Can you work these out from the model? Positions are in its coordinate system, mm. A direction names the side the tool comes from. Round coordinates to 2 decimals unless told otherwise and drop trailing zeros. Write each loop counter-clockwise with the first axis right and the second up, starting at its lowest first coordinate (ties: lowest second). Pieces come first, ordered by that corner, then holes.
Q1. We'd pull the mould along X, two halves only. Please class faces 5 (the cylindrical face through (1.4, -13.294, 613.956)), 6 (the flat face through (-70, 105, 629)), 7 (the flat face through (-50, 105, 629)): +X half, -X half, draft (parallel to the pull), parting line (faces both ways), or undercut.
Q2. I'm going to push flat-ended pins straight in: pin 1 Ø6 at (x, z) = (-34.5, 194) entering from +Y; pin 2 Ø20.5 at (x, y) = (-35, -665.5) entering from -Z; pin 3 Ø1 at (x, z) = (17.5, 164.5) entering from -Y; pin 4 Ø23.5 at (x, y) = (35, 665.5) entering from +Z. Where does each tip first touch, or does it pass through?
Q3. Please list where these lines run through material, in increasing order: line 1 along X through (y, z) = (-665.5, 37.75); line 2 along Y through (x, z) = (35, 29); line 3 along Y through (x, z) = (-35, 32).
Q4. If we section it at C-C (y = 373): Please give me the cut outline in (x, z), plus the area to 3 significant figures.
Q5. For faces 1 (the flat face through (50, -105, 629)), 2 (the flat face through (-1, 664, 45)), 3 (the flat face through (70, -105, 629)), 4 (the cylindrical face through (-84.79, 13.31, 633.96)), which set-ups out of +Z, -Z, +X, -X, +Y, -Y let a thin tool reach every point of the face, with its end or its side?
Q6. If we section it at B-B (z = 216): Please give me the cut outline in (x, y).
Q7. If we section it at D-D (z = 82.5): Please give me the cut outline in (x, y).
from build123d import *

# Parameters (mm, degrees)
F1_DEPTH  = 100
F4_DEPTH  = 20
F7_DEPTH  = 20
F8_W      = 200
F8_H      = 81.5832222524
F9_DEPTH  = 30
F10_R     = 9
F11_DEPTH = 672.101


with BuildPart() as f1:
    # F0 (on Right) → F1 (new body, symmetric)
    with BuildSketch(Plane.YZ):
        with BuildLine():
            ThreePointArc((-613.9167777476, 15), (0, 614.1), (613.9167777476, 15))
            Line((613.9167777476, 15), (633.9225583618, 15))
            ThreePointArc((633.9225583618, 15), (0, 634.1), (-633.9225583618, 15))
            Line((-633.9225583618, 15), (-613.9167777476, 15))
        make_face()
    extrude(amount=F1_DEPTH, both=True)

    # F3 (on offset) → F4 (join)
    with BuildSketch(Plane.YZ.offset(70)):
        with BuildLine():
            ThreePointArc((-633.9225583618, 15), (0, 634.1), (633.9225583618, 15))
            Line((633.9225583618, 15), (686.9362488616, 15))
            ThreePointArc((686.9362488616, 15), (0, 687.1), (-686.9362488616, 15))
            Line((-686.9362488616, 15), (-633.9225583618, 15))
        make_face()
    extrude(amount=-F4_DEPTH)

    # F6 (on offset) → F7 (join)
    with BuildSketch(Plane(origin=(-70, 0, 0), x_dir=(0, -1, 0), z_dir=(-1, 0, 0))):
        with BuildLine():
            Line((-686.9362488616, 15), (-633.9225583618, 15))
            ThreePointArc((-633.9225583618, 15), (0, 634.1), (633.9225583618, 15))
            Line((633.9225583618, 15), (686.9362488616, 15))
            ThreePointArc((686.9362488616, 15), (0, 687.1), (-686.9362488616, 15))
        make_face()
    extrude(amount=-F7_DEPTH)

    # F8 (on face) → F9 (join)
    with BuildSketch(Plane(origin=(0, 0, 15), x_dir=(1, 0, 0), z_dir=(0, 0, -1))):
        with Locations((0, -654.7083888738)):
            Rectangle(F8_W, F8_H)
        Polygon((-100, 695.5), (-100, 633.9225583618), (-70, 633.9225583618), (-70, 686.9362488616), (-50, 686.9362488616), (-50, 633.9225583618), (50, 633.9225583618), (50, 686.9362488616), (70, 686.9362488616), (70, 633.9225583618), (100, 633.9225583618), (100, 695.5), align=None)
        Polygon((-100, 633.9225583618), (-100, 613.9167777476), (100, 613.9167777476), (100, 633.9225583618), (70, 633.9225583618), (70, 686.9362488616), (50, 686.9362488616), (50, 633.9225583618), (-50, 633.9225583618), (-50, 686.9362488616), (-70, 686.9362488616), (-70, 633.9225583618), align=None)
    extrude(amount=-F9_DEPTH)

    # F10 (on face) → F11 (cut, through all)
    with BuildSketch(Plane(origin=(0, 0, 15), x_dir=(1, 0, 0), z_dir=(0, 0, -1))):
        with Locations((-35, 665.5)):
            Circle(F10_R)
        with Locations((35, 665.5)):
            Circle(F10_R)
        with Locations((-35, -665.5)):
            Circle(F10_R)
        with Locations((35, -665.5)):
            Circle(F10_R)
    extrude(amount=-F11_DEPTH, mode=Mode.SUBTRACT)


solid = f1.part
A:
1. face 5: draft
1. face 6: -X half
1. face 7: undercut
2. pin 1: stops at y = 604.65
2. pin 2: stops at z = 15
2. pin 3: stops at y = -612.52
2. pin 4: stops at z = 45
3. line 1: x = -100 to -44, -26 to 26, 44 to 100
3. line 2: y = -695.5 to -674.5, -656.5 to -613.41, 613.41 to 656.5, 674.5 to 695.5
3. line 3: y = -695.5 to -674.5, -656.5 to -613.27, 613.27 to 656.5, 674.5 to 695.5
4. outline: (-100, 487.84) - (100, 487.84) - (100, 512.79) - (70, 512.79) - (70, 577.04) - (50, 577.04) - (50, 512.79) - (-50, 512.79) - (-50, 577.04) - (-70, 577.04) - (-70, 512.79) - (-100, 512.79) - close
4. area: 7,560 mm2
5. face 1: +Z
5. face 2: +Z, +Y
5. face 3: +Z, +X
5. face 4: +Z, -X
6. outline: (-100, -596.18) - (-70, -596.18) - (-70, -652.27) - (-50, -652.27) - (-50, -596.18) - (50, -596.18) - (50, -652.27) - (70, -652.27) - (70, -596.18) - (100, -596.18) - (100, -574.86) - (-100, -574.86) - close; (-100, 574.86) - (100, 574.86) - (100, 596.18) - (70, 596.18) - (70, 652.27) - (50, 652.27) - (50, 596.18) - (-50, 596.18) - (-50, 652.27) - (-70, 652.27) - (-70, 596.18) - (-100, 596.18) - close
7. outline: (-100, -628.71) - (-70, -628.71) - (-70, -682.13) - (-50, -682.13) - (-50, -628.71) - (50, -628.71) - (50, -682.13) - (70, -682.13) - (70, -628.71) - (100, -628.71) - (100, -608.53) - (-100, -608.53) - close; (-100, 608.53) - (100, 608.53) - (100, 628.71) - (70, 628.71) - (70, 682.13) - (50, 682.13) - (50, 628.71) - (-50, 628.71) - (-50, 682.13) - (-70, 682.13) - (-70, 628.71) - (-100, 628.71) - close
